Autodesk Inventor part; units mm, degrees
ref_plane "YZ Plane" through (0, 0, 0) normal (1, 0, 0) x (0, 1, 0)
ref_plane "XZ Plane" through (0, 0, 0) normal (0, 1, 0) x (-1, 0, 0)
ref_plane "XY Plane" through (0, 0, 0) normal (0, 0, 1) x (1, 0, 0)
sketch "Sketch1" plane through (0, 0, 0) normal (0, 1, 0) x (-1, 0, 0)
  line L0 (0.5, 41) -> (12.5, 49)
  line L1 (0.5, 41) -> (12.5, 49)
  line L2 (12.5, 49) -> (11.9453, 49.8321)
  line L3 (11.9453, 49.8321) -> (-0.0547, 41.8321)
  arc A0 (-0.0547, 41.8321) -> (-0.5, 41) centre (0.5, 41) ccw
  line L4 (0.5, 41) -> (0.5, 0)
  line L5 (0.5, 0) -> (-0.5, 0)
  line L6 (-0.5, 0) -> (-0.5, 41)
  line L7 (0.5, -41) -> (12.5, -49)
  line L8 (12.5, -49) -> (11.9453, -49.8321)
  line L9 (11.9453, -49.8321) -> (-0.0547, -41.8321)
  arc A1 (-0.5, -41) -> (-0.0547, -41.8321) centre (0.5, -41) ccw
  line L10 (0.5, -41) -> (0.5, 0)
  line L11 (-0.5, 0) -> (-0.5, -41)
  point P0 (0, 0)
  dimension "d0" = 1
  dimension "d4" = 1
extrude "Extrusion1" add sketch "Sketch1" along normal blind 52
sketch "Sketch2" plane through (-0.5, 0, -41) normal (-1, 0, 0) x (0, 0, 1)
  circle A0 centre (15.8425, 26.5) radius 1.5
  circle A1 centre (66.1575, 26.5) radius 1.5
  line L0 (15.8425, 26.5) -> (15.8425, 0)
  line L1 (82, 0) -> (0, 0)
  line L2 (66.1575, 26.5) -> (66.1575, 0)
  line L3 (15.8425, 0) -> (20.8425, 0)
  line L4 (66.1575, 0) -> (71.1575, 0)
  line L5 (71.1575, 0) -> (61.1575, 0)
  line L6 (61.1575, 0) -> (61.1575, 10)
  line L7 (61.1575, 10) -> (71.1575, 10)
  line L8 (71.1575, 10) -> (71.1575, 0)
  line L9 (20.8425, 0) -> (10.8425, 0)
  line L10 (10.8425, 0) -> (10.8425, 10)
  line L11 (10.8425, 10) -> (20.8425, 10)
  line L12 (20.8425, 10) -> (20.8425, 0)
  dimension "d10" = 3
  dimension "d11" = 3
  dimension "d14" = 5
  dimension "d15" = 5
  dimension "d16" = 10
  dimension "d17" = 10
  dimension "d18" = 10
  dimension "d19" = 10
extrude "Extrusion2" cut sketch "Sketch2" against normal blind 1 contours A0 | A1
extrude "Extrusion3" cut sketch "Sketch2" against normal blind 1 contours L6 L7 L2 L1 | L11 L12 L1 L0 | L0 L1 L10 L11 | L2 L7 L8 L1
fillet "Fillet1" radius 5 4 edges at (-12.2226, 0, 49.416) (-12.2226, 52, 49.416) (-12.2226, 52, -49.416) (-12.2226, 0, -49.416)
properties part number "podpera_deska_rameno"
For this review, take the finished solid that the model builds, in its own axes (mm). A direction names the side the tool comes from. Coordinates: 2 decimals unless noted, no trailing zeros. Loops run counter-clockwise (first coordinate to the right, second up) from the corner with the lowest first, then second, coordinate; pieces in that order, holes last. Notation, with made-up numbers: (82.5, 17) -> (129.5, 17) arc R23 ccw to (129.5, 34) -> close; hole circle Ø7 at (46, 56). An arc over 180 degrees is marked (long way). Return JSON: item names as keys, results as strings. Group by question number.
(1) Consider section C-C, the plane z = -28.5. Give the boundary of the cut face in (x, y).
(2) For pin 1 Ø1.1 at (x, y) = (0, 6.5) entering from +Z; pin 2 Ø5 at (x, y) = (-11, 41) entering from -Z; pin 3 Ø4 at (x, z) = (-2, -20.5) entering from -Y; pin 4 Ø1.1 at (x, z) = (0, 24) entering from -Y, all flat-tipped, find the tip position at first contact; note any pin that passes through.
(3) Consider section D-D, the plane z = -1. Give the boundary of the cut face in (x, y), plus the area to 3 significant figures.
(4) Mouldability with a two-part tool opening along Y and no side actions: class faces 3 (the flat face through (-6.416, 25.636, -44.944)), 4 (the cylindrical face through (-0.007, 27.987, -25.353)), 5 (the cylindrical face through (-10.97, 50.57, 48.59)) as pulls with the +Y half, pulls with the -Y half, needs draft (parallel to the pull), parting line crosses it, or undercut.
(5) To check wall thickness, follow L1, parallel to Z at x = 0.05, y = 26.5; L2, parallel to Z at x = -0.2, y = 26.5; L3, parallel to X at y = 42.5, z = 37. State the ranges of each line that lie inside material, in increasing order.
(6) Consider section A-A, the plane x = -6.5. Give the boundary of the cut face in (y, z).
(7) Consider section B-B, the plane y = 26.5. Give the boundary of the cut face in (x, z).
(8) Tool access review of faces 1 (the flat face through (-6.03, 25.64, 45.89)), 2 (the flat face through (-6.416, 25.636, 44.944)): name each direction out of +Z, -Z, +X, -X, +Y, -Y from which nothing blocks a thin tool from reaching the whole face with its end or side.
Results below:
{
 "1": {"outline": "(-0.5, 10) -> (0.5, 10) -> (0.5, 52) -> (-0.5, 52) -> close"},
 "2": {"pin 1": "stops at z = 42.24", "pin 2": "stops at z = -49.83", "pin 3": "stops at y = 0", "pin 4": "stops at y = 10"},
 "3": {"outline": "(-0.5, 0) -> (0.5, 0) -> (0.5, 52) -> (-0.5, 52) -> close", "area": "52.0 mm2"},
 "4": {"face 3": "needs draft", "face 4": "undercut", "face 5": "pulls with the +Y half"},
 "5": {"L1": "z = -41.84 to -26.66, -23.66 to 23.66, 26.66 to 41.84", "L2": "z = -42 to -26.66, -23.66 to 23.66, 26.66 to 42", "L3": "x = -0.5 to 0.5"},
 "6": {"outline": "(0, -46.2) -> (52, -46.2) -> (52, -45) -> (0, -45) -> close; (0, 45) -> (52, 45) -> (52, 46.2) -> (0, 46.2) -> close"},
 "7": {"outline": "(-12.5, -49) -> (-11.95, -49.83) -> (0.05, -41.83) arc R1 ccw to (0.5, -41) -> (0.5, -26.66) -> (-0.5, -26.66) -> (-0.5, -41) -> close; (-12.5, 49) -> (-0.5, 41) -> (-0.5, 26.66) -> (0.5, 26.66) -> (0.5, 41) arc R1 ccw to (0.05, 41.83) -> (-11.95, 49.83) -> close; (-0.5, -23.66) -> (0.5, -23.66) -> (0.5, 23.66) -> (-0.5, 23.66) -> close"},
 "8": {"face 1": "+Z, +X, +Y, -Y", "face 2": "-X, +Y, -Y"}
}
